Study the drawing (mm; zero at the part's minimum x, y, z) and answer. Coordinates: 2 decimals unless noted, no trailing zeros. Order: outer loops, then holes, each group sorted by start corner. A loop starts at its lowest first (then second) coordinate and runs counter-clockwise, first axis right, second up. Notation, with made-up numbers: (70.5, 68) -> (78.5, 68) arc R12 cw to (78.5, 91) -> close; hole circle Ø8 at (77, 13). An arc over 180 degrees is marked (long way). Answer as CSV lines item,"result". Start each with the question number.
Item 1: This flat-tipped pin is pushed along its axis until it touches: pin 1 Ø2 at (x, z) = (102.5, 205.5) entering from -Y. Where does it stop, or does it pass through?
Item 2: Section C-C (x = 157.5) is taken. Write down the section's boundary in (y, z), then the cut area to 3 significant figures.
Item 3: Section B-B (y = 3) is taken. Write down the section's boundary in (x, z), then the cut area to 3 significant figures.
Item 4: Section A-A (z = 40) is taken. Write down the section's boundary in (x, y), then the cut area to 3 significant figures.
Item 5: Straight lines are drawn through the part: L1, parallel to X at y = 6.5, z = 40; L2, parallel to X at y = 5.25, z = 30.5; L3, parallel to Z at x = 50, y = 6.25. For each, find the intervals that lie inside material, in ascending order.
Item 6: Section D-D (x = 250.5) is taken. Write down the section's boundary in (y, z) (3 decimals), then the cut area to 3 significant figures.
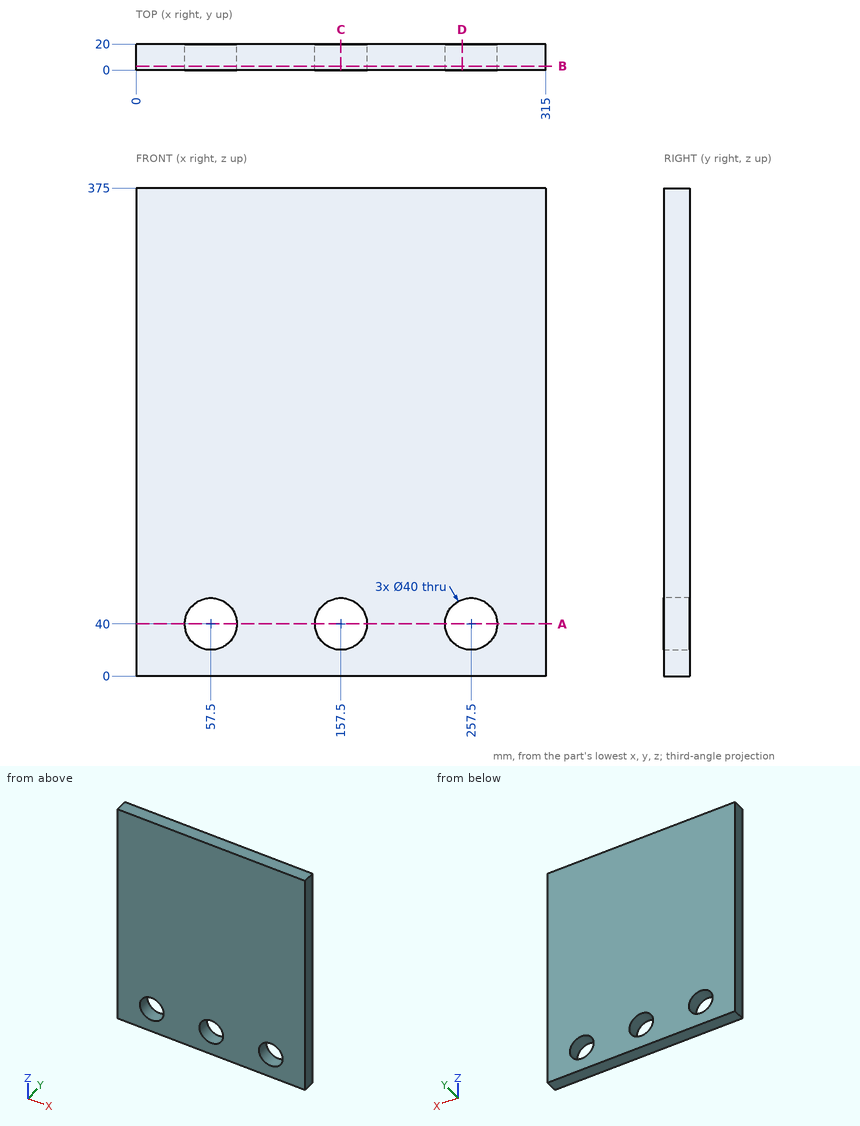
Checked values:
1,pin 1,"stops at y = 0"
2,outline,"(0, 0) -> (20, 0) -> (20, 20) -> (0, 20) -> close; (0, 60) -> (20, 60) -> (20, 375) -> (0, 375) -> close"
2,area,"6,700 mm^2"
3,outline,"(0, 0) -> (315, 0) -> (315, 375) -> (0, 375) -> close; hole circle Ø40 at (57.5, 40); hole circle Ø40 at (157.5, 40); hole circle Ø40 at (257.5, 40)"
3,area,"114,000 mm^2"
4,outline,"(0, 0) -> (37.5, 0) -> (37.5, 20) -> (0, 20) -> close; (77.5, 0) -> (137.5, 0) -> (137.5, 20) -> (77.5, 20) -> close; (177.5, 0) -> (237.5, 0) -> (237.5, 20) -> (177.5, 20) -> close; (277.5, 0) -> (315, 0) -> (315, 20) -> (277.5, 20) -> close"
4,area,"3,900 mm^2"
5,L1,"x = 0 to 37.5, 77.5 to 137.5, 177.5 to 237.5, 277.5 to 315"
5,L2,"x = 0 to 39.9, 75.1 to 139.9, 175.1 to 239.9, 275.1 to 315"
5,L3,"z = 0 to 21.46, 58.54 to 375"
6,outline,"(0, 0) -> (20, 0) -> (20, 21.265) -> (0, 21.265) -> close; (0, 58.735) -> (20, 58.735) -> (20, 375) -> (0, 375) -> close"
6,area,"6,750 mm^2"
